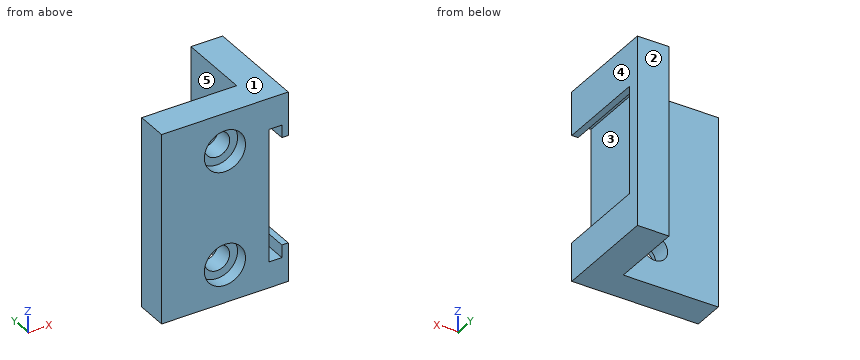
from build123d import *

# Parameters (mm, degrees)
SALIENTE_EXTRUIR1_DEPTH = 30
CORTAR_EXTRUIR1_START   = -14.5
CORTAR_EXTRUIR1_DEPTH   = 14.5
CORTAR_EXTRUIR2_REACH   = 39.286
CROQUIS3_R              = 2
CROQUIS4_R              = 3.25
CORTAR_EXTRUIR3_DEPTH   = 2
CROQUIS5_W              = 5
CROQUIS5_H              = 30
SALIENTE_EXTRUIR2_DEPTH = 2


# Read off the part's stored shape, not the designer's step: Cortar-Extruir1
with BuildPart() as part:
    # Croquis1 → Saliente-Extruir1 (new body)
    with BuildSketch(Plane.XY):
        Polygon((20, 0), (20, 14.5), (15, 14.5), (15, 5), (0, 5), (0, 0), align=None)
    extrude(amount=SALIENTE_EXTRUIR1_DEPTH)

    # Cortar-Extruir1 outline → Cortar-Extruir1 (cut)
    with BuildSketch(Plane(origin=(0, 14.5, 0), x_dir=(1, 0, 0), z_dir=(0, 1, 0)).offset(CORTAR_EXTRUIR1_START)):
        Polygon((20, -23.1), (20, -6.1), (19, -6.1), (19, -4.1), (16.96, -4.1), (16.96, -25.1), (19, -25.1), (19, -23.1), align=None)
    extrude(amount=CORTAR_EXTRUIR1_DEPTH, mode=Mode.SUBTRACT)

    # Croquis3 → Cortar-Extruir2 (cut, up to next)
    with BuildSketch(Plane(origin=(0, 5, 0), x_dir=(1, 0, 0), z_dir=(0, 1, 0)), mode=Mode.PRIVATE) as cortar_extruir2_sk1:
        with Locations(Location((10, -6, 0), (0, 0, 270))):
            Circle(CROQUIS3_R)
    cortar_extruir2_tool1 = extrude(cortar_extruir2_sk1.sketch, amount=-CORTAR_EXTRUIR2_REACH, mode=Mode.PRIVATE) & part.part
    # Croquis3 → Cortar-Extruir2 (cut, up to next)
    with BuildSketch(Plane(origin=(0, 5, 0), x_dir=(1, 0, 0), z_dir=(0, 1, 0)), mode=Mode.PRIVATE) as cortar_extruir2_sk2:
        with Locations(Location((10, -24, 0), (0, 0, 270))):
            Circle(CROQUIS3_R)
    cortar_extruir2_tool2 = extrude(cortar_extruir2_sk2.sketch, amount=-CORTAR_EXTRUIR2_REACH, mode=Mode.PRIVATE) & part.part
    add(cortar_extruir2_tool1.solids().sort_by_distance((10, 5, 6))[0], mode=Mode.SUBTRACT)
    add(cortar_extruir2_tool2.solids().sort_by_distance((10, 5, 24))[0], mode=Mode.SUBTRACT)

    # Croquis4 → Cortar-Extruir3 (cut)
    with BuildSketch(Plane.XZ):
        with Locations(Location((10, 24, 0), (0, 0, 270))):
            Circle(CROQUIS4_R)
        with Locations(Location((10, 6, 0), (0, 0, 90))):
            Circle(CROQUIS4_R)
    extrude(amount=-CORTAR_EXTRUIR3_DEPTH, mode=Mode.SUBTRACT)

    # Croquis5 → Saliente-Extruir2 (add)
    with BuildSketch(Plane(origin=(0, 14.5, 0), x_dir=(1, 0, 0), z_dir=(0, 1, 0))):
        with Locations((17.5, -15)):
            Rectangle(CROQUIS5_W, CROQUIS5_H)
    extrude(amount=SALIENTE_EXTRUIR2_DEPTH)


solid = part.part
Design review of the part built by this model. Coordinates are the model's own, in mm. Face numbers are marked on the shaded views. A direction names the side the tool comes from. Round coordinates to 2 decimals unless told otherwise and drop trailing zeros. Loops run counter-clockwise (first coordinate to the right, second up) from the corner with the lowest first, then second, coordinate; pieces in that order, holes last. Notation, with made-up numbers: (84, -28.75) - (123, -28.75) arc R16 cw to (123, -5.75) - close; hole circle Ø8 at (80, -31.75). An arc over 180 degrees is marked (long way). One line per item, written item: value. Start each with the question number.
1) Consider section A-A on x = 10. Give the boundary of the cut face in (y, z).
2) Consider section B-B on y = 1.5. Give the boundary of the cut face in (x, z).
3) For the marked faces 4 and 5, list the 3-axis set-ups (+Z, -Z, +X, -X, +Y, -Y) from which the entire face can be reached by the end or side of a thin tool; tool diameter is ignored.
4) Consider section C-C on z = 24. Give the boundary of the cut face in (x, y).
5) Draft analysis for pull direction Z (two halves, no side actions). For the marked faces 1, 2 and 3, state which applies: +Z half, -Z half, draft (parallel to the pull), parting line (faces both ways), or undercut.
6) Insertion check: pin 1 Ø2 at (x, z) = (11.5, 6.5) entering from -Y; pin 2 Ø7 at (x, z) = (11, 24.5) entering from -Y; pin 3 Ø7 at (y, z) = (8, 17.5) entering from +X; pin 4 Ø5 at (y, z) = (12, 4.5) entering from -X. Each pin has a flat end and moves straight along its axis. Give the tip position at first contact, or say it passes through.
7) Consider section D-D on z = 14. Give the boundary of the cut face in (x, y).
8) To check wall thickness, follow L1, parallel to X at y = 3.7, z = 24; L2, parallel to X at y = 1.25, z = 24; L3, parallel to Y at x = 9.25, z = 20.5. State the ranges of each line that lie inside material, in increasing order. Write a range as from..to.
Reported:
1. outline: (0, 0) - (5, 0) - (5, 4) - (2, 4) - (2, 2.75) - (0, 2.75) - close; (0, 9.25) - (2, 9.25) - (2, 8) - (5, 8) - (5, 22) - (2, 22) - (2, 20.75) - (0, 20.75) - close; (0, 27.25) - (2, 27.25) - (2, 26) - (5, 26) - (5, 30) - (0, 30) - close
2. outline: (0, 0) - (20, 0) - (20, 6.1) - (19, 6.1) - (19, 4.1) - (16.96, 4.1) - (16.96, 25.1) - (19, 25.1) - (19, 23.1) - (20, 23.1) - (20, 30) - (0, 30) - close; hole circle Ø6.5 at (10, 6); hole circle Ø6.5 at (10, 24)
3. face 4: +Z, -Z, +X, +Y, -Y
3. face 5: +Z, -Z, -X, +Y
4. outline: (0, 0) - (6.75, 0) - (6.75, 2) - (8, 2) - (8, 5) - (0, 5) - close; (12, 2) - (13.25, 2) - (13.25, 0) - (16.96, 0) - (16.96, 14.5) - (19, 14.5) - (19, 0) - (20, 0) - (20, 16.5) - (15, 16.5) - (15, 5) - (12, 5) - close
5. face 1: +Z half
5. face 2: draft
5. face 3: undercut
6. pin 1: stops at y = 2
6. pin 2: stops at y = 0
6. pin 3: stops at x = 16.96
6. pin 4: stops at x = 15
7. outline: (0, 0) - (16.96, 0) - (16.96, 14.5) - (20, 14.5) - (20, 16.5) - (15, 16.5) - (15, 5) - (0, 5) - close
8. L1: x = 0..8, 12..16.96, 19..20
8. L2: x = 0..6.75, 13.25..16.96, 19..20
8. L3: y = 0..5
